For this review, take the finished solid that the model builds, in its own axes (mm). A direction names the side the tool comes from. Give positions to 0.01 mm unless a question says otherwise; leave off trailing zeros. Write each loop counter-clockwise with the first axis right and the second up, starting at its lowest first coordinate (ties: lowest second). Pieces come first, ordered by that corner, then holes.
1) Machinability: for faces 1 (the face through (11, 121, 35.824)), 2 (the face through (37, 121, -9.856)), 3 (the face through (51.818, 55, -19)), 4 (the face through (20, 0, 23)), 5 (the face through (11, -12, 35.301)), which of the approach directions +Z, -Z, +X, -X, +Y, -Y give a long, thin tool a straight path to every point of the face, cutting with its end or side? Answer none if there is none.
2) We need section C-C on x = 36. Give the boundary of the cut face in (y, z), and give its area (3 significant figures).
3) Draft analysis for pull direction X (two halves, no side actions). For faces 6 (the face through (20, 108, 23)), 7 (the face through (42.744, -12, 5)), 8 (the face through (29.924, -12, 5)), state which applies: pulls with the +X half, pulls with the -X half, needs draft (parallel to the pull), parting line crosses it, or undercut.
4) Wall thickness on line 1 along Z through (x, y) = (-3, -5.5); line 2 along Z through (x, y) = (-14, 24); line 3 along X through (y, z) = (14.5, -16.5): over which ranges is each line inside the solid? List them lowest first.
5) We need section A-A on x = -20. Give the boundary of the cut face in (y, z).
6) We need section B-B on z = 9.5. Give the boundary of the cut face in (x, y).
7) We need section D-D on y = 112. Give the boundary of the cut face in (x, z), and give its area (3 significant figures).
8) For P1, Ø8, axis at x = 54.5, y = 123.5, coming from the -Z side; P2, Ø3, axis at x = 39.5, y = 95, coming from the +Z side; P3, Ø20, axis at x = 7.5, y = 123.5, coming from the +Z side; P4, Ø7.5, axis at y = 121, z = 13, coming from the +X side, all flat-tipped, find the tip position at first contact; note any pin that passes through.
from build123d import *

# Parameters (mm, degrees)
F1_DEPTH = 133
F0_W     = 12.819961
F0_H     = 30.998608
F2_DEPTH = 25
F4_W     = 13.766533
F4_H     = 30.66182
F5_DEPTH = 25


with BuildPart() as f1:
    # F0 (on Front) → F1 (new body)
    with BuildSketch(Plane.XZ):
        Polygon((29.924046, -10.552499), (-39.667495, -10.552499), (-39.667495, 20.446109), (-39.667495, 35.30141), (-39.667495, 121.849649), (-59.0625, 121.849649), (-59.0625, -10.552499), (-59.0625, -26.9325), (51.817503, -26.9325), (51.817503, -10.552499), (42.744007, -10.552499), align=None)
    extrude(amount=-F1_DEPTH)

    # F0 (on Front) → F2 (join)
    with BuildSketch(Plane.XZ):
        Polygon((29.924046, -10.552499), (-39.667495, -10.552499), (-39.667495, 20.446109), (-39.667495, 35.30141), (-39.667495, 121.849649), (-59.0625, 121.849649), (-59.0625, -10.552499), (-59.0625, -26.9325), (51.817503, -26.9325), (51.817503, -10.552499), (42.744007, -10.552499), align=None)
        with Locations((36.334026, 4.946805)):
            Rectangle(F0_W, F0_H)
        Polygon((-39.667495, 35.30141), (-39.667495, 20.446109), (29.924046, 20.446109), (42.744007, 20.446109), (59.634183, 20.446109), (59.634183, 35.30141), align=None)
    extrude(amount=F2_DEPTH)

    # F4 (on offset) → F5 (join)
    with BuildSketch(Plane.XZ.offset(-133)):
        Polygon((59.915699, 20.806234), (59.915699, 35.824269), (-42.081788, 35.824269), (-42.081788, 20.806234), (29.879631, 20.806234), (43.646164, 20.806234), align=None)
        with Locations((36.762898, 5.475324)):
            Rectangle(F4_W, F4_H)
    extrude(amount=F5_DEPTH)


solid = f1.part
Results list:
1. face 1: +Z, +X, +Y, -Y
1. face 2: +X, +Y
1. face 3: -Z, +X, +Y, -Y
1. face 4: +Z, +X
1. face 5: +Z, +X, -Y
2. outline: (-25, -26.93) - (133, -26.93) - (133, -10.55) - (0, -10.55) - (0, 35.3) - (-25, 35.3) - close; (108, -9.86) - (133, -9.86) - (133, 35.82) - (108, 35.82) - close
2. area: 4,880 mm2
3. face 6: needs draft
3. face 7: pulls with the +X half
3. face 8: undercut
4. line 1: z = -26.93 to -10.55, 20.45 to 35.3
4. line 2: z = -26.93 to -10.55
4. line 3: x = -59.06 to 51.82
5. outline: (-25, -26.93) - (133, -26.93) - (133, -10.55) - (-25, -10.55) - close; (-25, 20.45) - (0, 20.45) - (0, 35.3) - (-25, 35.3) - close; (108, 20.81) - (133, 20.81) - (133, 35.82) - (108, 35.82) - close
6. outline: (-59.06, -25) - (-39.67, -25) - (-39.67, 133) - (-59.06, 133) - close; (29.88, 108) - (43.65, 108) - (43.65, 133) - (29.88, 133) - close; (29.92, -25) - (42.74, -25) - (42.74, 0) - (29.92, 0) - close
7. outline: (-59.06, -26.93) - (51.82, -26.93) - (51.82, -10.55) - (-39.67, -10.55) - (-39.67, 20.81) - (29.88, 20.81) - (29.88, -9.86) - (43.65, -9.86) - (43.65, 20.81) - (59.92, 20.81) - (59.92, 35.82) - (-39.67, 35.82) - (-39.67, 121.85) - (-59.06, 121.85) - close
7. area: 6,300 mm2
8. P1: stops at z = -26.93
8. P2: stops at z = -10.55
8. P3: stops at z = 35.82
8. P4: stops at x = 43.65
